Model file for the job. Use its own axes, mm. A direction names the side the tool comes from. Round coordinates to 2 decimals unless told otherwise and drop trailing zeros. Order: outer loops, then holes, each group sorted by start corner. A loop starts at its lowest first (then second) coordinate and runs counter-clockwise, first axis right, second up. Notation, with made-up numbers: (-34.75, 81) - (17.25, 81) arc R27 ccw to (17.25, 117) - close; hole circle Ø8 at (12, 1). An arc over 180 degrees is marked (long way). Put each result on its own line as item: value. Start each with the question number.
Item 1: Mould opens along Z. For faces 5 (the face through (-10, 7, -33)), 6 (the face through (-12, 7, -36)), 7 (the face through (3.954, 3.16, 0.878)) say: pulls with the +Z half, pulls with the -Z half, needs draft (parallel to the pull), parting line crosses it, or undercut.
Item 2: Saw through at D-D on y = 1.75. List the corners of the cut face in (x, z), plus the area to 3 significant figures.
Item 3: Saw through at C-C on x = 0. State how many separate pieces and enclosed holes the cut face has, plus the area to 3 significant figures.
Item 4: Probe probe 1 along Y at (x, z) = (0, -26.4); probe 2 along X at (y, z) = (10, -28.3); probe 3 along Z at (x, y) = (2.75, 13.25). List the from-to ranges inside material, lowest first.
Item 5: Saw through at A-A on z = -29. List the corners of the cut face in (x, y), plus the area to 3 significant figures.
Item 6: Saw through at B-B on y = 6. List the corners of the cut face in (x, z), plus the area to 3 significant figures.
Item 7: Pin check, flat tips, straight feed: pin 1 Ø4 at (y, z) = (3.5, -13.5) entering from -X; pin 2 Ø7.5 at (x, z) = (0, 0) entering from +Y; pin 3 Ø3 at (x, z) = (-7, 0.5) entering from +Y; pin 4 Ø1.5 at (x, y) = (-7, 11.5) entering from +Z. Stop position of each tip, or through.
Item 8: Which spindle directions (+Z, -Z, +X, -X, +Y, -Y) get a long thin tool onto all of the face, cutting with end or side? Do faces 1 (the face through (-10, 12, -25)), 2 (the face through (0, 6, -30)), 3 (the face through (-5, 15, -28)), 4 (the face through (-10, 3, -12)). Say none if no direction does.
```python
from build123d import *

# Parameters (mm, degrees)
BOSS_EXTRUDE1_DEPTH = 5
SKETCH2_W           = 25
SKETCH2_H           = 11
BOSS_EXTRUDE2_DEPTH = 10
SKETCH3_W           = 20
SKETCH3_H           = 6
CUT_EXTRUDE1_DEPTH  = 16
FILLET1_R           = 1.5
FILLET2_R           = 2.5
FILLET3_R           = 5
FILLET4_R           = 10


with BuildPart() as part:
    # Sketch1 → Boss-Extrude1 (new body)
    with BuildSketch(Plane(origin=(0, 5, 0), x_dir=(1, 0, 0), z_dir=(0, 1, 0))):
        with BuildLine():
            Line((10, 5.775897312), (10, 36))
            Line((10, 36), (-15, 36))
            Line((-15, 36), (-15, 25))
            Line((-15, 25), (-10, 16.339745962))
            Line((-10, 16.339745962), (-10, 5.775897312))
            Line((-10, 5.775897312), (-7.684618874, -2.224102688))
            ThreePointArc((-7.684618874, -2.224102688), (0, -8), (7.684618874, -2.224102688))
            Line((7.684618874, -2.224102688), (10, 5.775897312))
        make_face()
    extrude(amount=-BOSS_EXTRUDE1_DEPTH)

    # Sketch2 → Boss-Extrude2 (add)
    with BuildSketch(Plane(origin=(0, 5, 0), x_dir=(-1, 0, 0), z_dir=(0, 1, 0))):
        with Locations((2.5, -30.5)):
            Rectangle(SKETCH2_W, SKETCH2_H)
    extrude(amount=BOSS_EXTRUDE2_DEPTH)

    # Sketch3 → Cut-Extrude1 (cut, through all)
    with BuildSketch(Plane.XZ):
        with Locations((0, -33)):
            Rectangle(SKETCH3_W, SKETCH3_H)
    extrude(amount=-CUT_EXTRUDE1_DEPTH, mode=Mode.SUBTRACT)

    # Sketch6 → Ø8.1 (8.1) Diameter Hole1 (revolve, cut)
    with BuildSketch(Plane(origin=(0, 0, 0), x_dir=(0, 0, -1), z_dir=(1, 0, 0))):
        Polygon((0, 0), (0, 15), (4.05, 15), (4.05, 2.5), (4.719872981, 0), align=None)
    revolve(axis=Axis((0, -6.35, 0), (0, 1, 0)), mode=Mode.SUBTRACT)

    # Sketch4 → CBORE for M5 SBHCS1 (revolve, cut)
    with BuildSketch(Plane(origin=(0, 10, -25), x_dir=(0, -1, 0), z_dir=(1, 0, 0))):
        Polygon((0, 0), (0, 11), (2.65, 11), (2.65, 0.1), (5.25, 0.1), (5.25, 0), align=None)
    revolve(axis=Axis((0, 10, -18.65), (0, 0, -1)), mode=Mode.SUBTRACT)

    # Fillet1
    fillet1_edges = [part.edges().sort_by_distance(p)[0] for p in [
        (0, 5, 4.05),
    ]]
    fillet(fillet1_edges, radius=FILLET1_R)

    # Fillet2
    fillet2_edges = [part.edges().sort_by_distance(p)[0] for p in [
        (0, 2.5, 4.05),
    ]]
    fillet(fillet2_edges, radius=FILLET2_R)

    # Fillet3
    fillet3_edges = [part.edges().sort_by_distance(p)[0] for p in [
        (-8.30039053, 5, -25),
        (5.80039053, 5, -25),
    ]]
    fillet(fillet3_edges, radius=FILLET3_R)

    # Fillet4
    fillet4_edges = [part.edges().sort_by_distance(p)[0] for p in [
        (-10, 2.5, -5.775897312),
        (10, 2.5, -5.775897312),
    ]]
    fillet(fillet4_edges, radius=FILLET4_R)


solid = part.part
```
Results found:
1. face 5: needs draft
1. face 6: pulls with the -Z half
1. face 7: undercut
2. outline: (-15, -36) - (-10, -36) - (-10, -30) - (10, -30) - (10, -7.19) arc R10 ccw to (9.61, -4.41) - (7.68, 2.22) arc R8 ccw to (-7.68, 2.22) - (-9.61, -4.41) arc R10 ccw to (-10, -7.19) - (-10, -16.34) - (-15, -25) - close; hole circle Ø8.5 at (0, 0)
2. area: 711 mm²
3. separate pieces: 3
3. enclosed holes: 0
3. area: 170 mm²
4. probe 1: y = 0 to 7.35, 12.65 to 15
4. probe 2: x = -15 to -2.65, 2.65 to 10
4. probe 3: z = -30 to -25.1
5. outline: (-15, 0) - (10, 0) - (10, 15) - (-15, 15) - close; hole circle Ø5.3 at (0, 10)
5. area: 353 mm²
6. outline: (-15, -36) - (-10, -36) - (-10, -30) - (10, -30) - (10, -23) - (3.4, -23) - (3.4, -25.1) - (-3.4, -25.1) - (-3.4, -23) - (-13.85, -23) - (-15, -25) - close
6. area: 190 mm²
7. pin 1: stops at x = -10
7. pin 2: passes through
7. pin 3: stops at y = 5
7. pin 4: stops at z = -25
8. face 1: +Z, +X, -X, +Y
8. face 2: -Z, +X, +Y, -Y
8. face 3: +Z, -Z, +X, -X, +Y
8. face 4: +Z, -X, +Y, -Y
